For this review, take the finished solid that the model builds, in its own axes (mm). Face numbers are marked on the shaded views. Give positions to 0.01 mm unless a question says otherwise; leave off trailing zeros. Order: outer loops, then holes, each group sorted by start corner. A loop starts at its lowest first (then second) coordinate and runs counter-clockwise, first axis right, second up.
Item 1: Consider section C-C (z = 1.75). Give the boundary of the cut face in (x, y).
Item 2: For P1, Ø1.5, axis at y = 2.5, z = 1.5, coming from the -X side, flat-tipped, find the tip position at first contact; note if it passes through.
Item 3: Consider section A-A (y = 0). Give the boundary of the cut face in (x, z).
Item 4: For probe 1 along Y at (x, z) = (-7, 1.25); probe 2 along Z at (x, y) = (6, -2.75); probe 3 along X at (y, z) = (1.25, 1.85), list the stretches that pass through material, from the lowest coordinate up.
Item 5: Consider section D-D (y = -2.5). Give the boundary of the cut face in (x, z).
Item 6: Consider section B-B (x = 7). Give the boundary of the cut face in (y, z), plus the area to 3 significant figures.
Item 7: The part is to be moulded in two halves that separate along Y. For the marked faces 1 and 2, say which applies: released by +Y, released by -Y, zero draft, split by the parting line, or undercut.
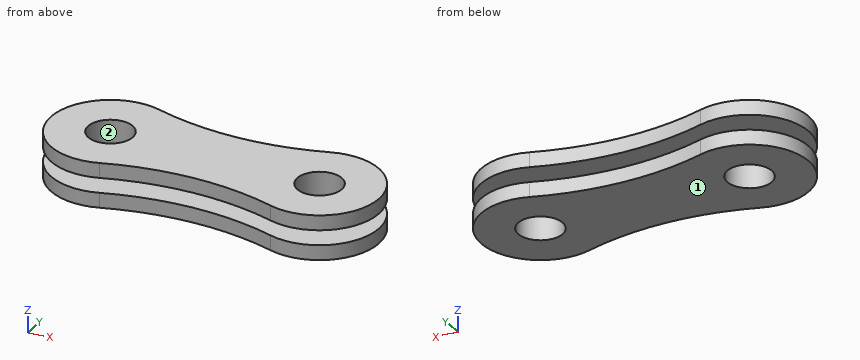
```python
from build123d import *

# Parameters (mm, degrees)
SKETCH1_R           = 1.5
BOSS_EXTRUDE1_DEPTH = 1
SKETCH2_R           = 2
SKETCH2_R_2         = 1.5
BOSS_EXTRUDE2_DEPTH = 2


with BuildPart() as part:
    # Sketch1 → Boss-Extrude1 (new body)
    with BuildSketch(Plane.XY):
        with BuildLine():
            ThreePointArc((-5.727272727, 3.792118839), (-11, 0), (-5.727272727, -3.792118839))
            ThreePointArc((-5.727272727, -3.792118839), (0, -2.856653615), (5.727272727, -3.792118839))
            ThreePointArc((5.727272727, -3.792118839), (11, 0), (5.727272727, 3.792118839))
            ThreePointArc((5.727272727, 3.792118839), (0, 2.856653615), (-5.727272727, 3.792118839))
        make_face()
        with Locations((-7, 0)):
            Circle(SKETCH1_R, mode=Mode.SUBTRACT)
        with Locations((7, 0)):
            Circle(SKETCH1_R, mode=Mode.SUBTRACT)
    boss_extrude1 = extrude(amount=BOSS_EXTRUDE1_DEPTH)

    # Sketch2 → Boss-Extrude2 (add)
    with BuildSketch(Plane.XY.offset(1)):
        with Locations((-7, 0)):
            Circle(SKETCH2_R)
        with Locations((-7, 0)):
            Circle(SKETCH2_R_2, mode=Mode.SUBTRACT)
        with Locations((7, 0)):
            Circle(SKETCH2_R)
        with Locations((7, 0)):
            Circle(SKETCH2_R_2, mode=Mode.SUBTRACT)
    extrude(amount=BOSS_EXTRUDE2_DEPTH)

    # Mirror1: Boss-Extrude1 across plane
    add(boss_extrude1.mirror(Plane.XY.offset(1.5)))


solid = part.part
```
Resolved:
1. outline: circle Ø4 at (-7, 0); circle Ø4 at (7, 0); hole circle Ø3 at (-7, 0); hole circle Ø3 at (7, 0)
2. P1: stops at x = -10.5
3. outline: (-11, 0) - (-8.5, 0) - (-8.5, 3) - (-11, 3) - (-11, 2) - (-9, 2) - (-9, 1) - (-11, 1) - close; (-5.5, 0) - (5.5, 0) - (5.5, 3) - (-5.5, 3) - close; (8.5, 0) - (11, 0) - (11, 1) - (9, 1) - (9, 2) - (11, 2) - (11, 3) - (8.5, 3) - close; hole (-5, 1) - (5, 1) - (5, 2) - (-5, 2) - close
4. probe 1: y = -2 to -1.5, 1.5 to 2
4. probe 2: z = 0 to 1, 2 to 3
4. probe 3: x = -8.56 to -7.83, -6.17 to -5.44, 5.44 to 6.17, 7.83 to 8.56
5. outline: (-10.12, 0) - (10.12, 0) - (10.12, 1) - (-10.12, 1) - close; (-10.12, 2) - (10.12, 2) - (10.12, 3) - (-10.12, 3) - close
6. outline: (-4, 0) - (-1.5, 0) - (-1.5, 3) - (-4, 3) - (-4, 2) - (-2, 2) - (-2, 1) - (-4, 1) - close; (1.5, 0) - (4, 0) - (4, 1) - (2, 1) - (2, 2) - (4, 2) - (4, 3) - (1.5, 3) - close
6. area: 11.0 mm2
7. face 1: zero draft
7. face 2: undercut
